For this review, take the finished solid that the model builds, in its own axes (mm). A direction names the side the tool comes from. Coordinates: 2 decimals unless noted, no trailing zeros. Loops run counter-clockwise (first coordinate to the right, second up) from the corner with the lowest first, then second, coordinate; pieces in that order, holes last.
1. Machinability: for faces 4 (the face through (2, -5, 5)), 5 (the face through (2, 7, 0)), which of the approach directions +Z, -Z, +X, -X, +Y, -Y give a long, thin tool a straight path to every point of the face, cutting with its end or side? Answer none if there is none.
2. Clearance check with flat-ended pins moving along their axes: P1, Ø2.5, axis at x = 12, z = 5, coming from the +Y side; P2, Ø4, axis at y = 1, z = 8.5, coming from the -X side; P3, Ø1.8, axis at x = 12, z = 5, coming from the -Y side. State where each tip first meets the part, or that it passes through.
3. Take a section at D-D, the plane y = -4.25. State the section outline as (x, z) points.
4. Take a section at A-A, the plane x = 3. State the section outline as (y, z) points.
5. Mouldability with a two-part tool opening along Y and no side actions: class faces 1 (the face through (13, 0, 5)), 2 (the face through (2, -10, 5)), 3 (the face through (3, 10, 5)) as pulls with the +Y half, pulls with the -Y half, needs draft (parallel to the pull), parting line crosses it, or undercut.
6. To check wall thickness, follow probe 1 along X at (y, z) = (8.1, 5); probe 2 along Y at (x, z) = (12.75, 6.25); probe 3 along Z at (x, y) = (12, -6.45). State the ranges of each line that lie inside material, in increasing order.
7. Take a section at C-C, the plane y = -7.5. State the section outline as (x, z) points, then the cut area to 3 significant figures.
8. Take a section at B-B, the plane z = 7. State the section outline as (x, y) points.
```python
from build123d import *

# Parameters (mm, degrees)
F0_W     = 2
F0_H     = 10
F1_DEPTH = 10
F3_DEPTH = 20


with BuildPart() as f1:
    # F0 (on Top) → F1 (new body)
    with BuildSketch(Plane.XY):
        Polygon((-1, 5), (0, 5), (1, 5), (13, 5), (15, 5), (15, 10), (-10, 10), (-10, 5), align=None)
        Polygon((1, -5), (0, -5), (-1, -5), (-10, -5), (-10, -10), (15, -10), (15, -5), (13, -5), align=None)
        with Locations((14, 0)):
            Rectangle(F0_W, F0_H)
    extrude(amount=F1_DEPTH)

    # F2 (on face) → F3 (cut)
    with BuildSketch(Plane.XZ.offset(10)):
        with BuildLine():
            ThreePointArc((12, 4), (12.707107, 4.292893), (13, 5))
            ThreePointArc((13, 5), (11.292893, 5.707107), (12, 4))
        make_face()
        with BuildLine():
            ThreePointArc((-7, 4), (-6.292893, 4.292893), (-6, 5))
            ThreePointArc((-6, 5), (-7.707107, 5.707107), (-7, 4))
        make_face()
    extrude(amount=-F3_DEPTH, mode=Mode.SUBTRACT)


solid = f1.part
```
Results list:
1. face 4: +Z, -Z, -X
1. face 5: -Z, +X, -X, +Y, -Y
2. P1: stops at y = 10
2. P2: stops at x = 13
2. P3: passes through
3. outline: (13, 0) - (15, 0) - (15, 10) - (13, 10) - close
4. outline: (-10, 0) - (-5, 0) - (-5, 10) - (-10, 10) - close; (5, 0) - (10, 0) - (10, 10) - (5, 10) - close
5. face 1: undercut
5. face 2: pulls with the -Y half
5. face 3: pulls with the +Y half
6. probe 1: x = -10 to -8, -6 to 11, 13 to 15
6. probe 2: y = -10 to -5, 5 to 10
6. probe 3: z = 0 to 4, 6 to 10
7. outline: (-10, 0) - (15, 0) - (15, 10) - (-10, 10) - close; hole circle Ø2 at (-7, 5); hole circle Ø2 at (12, 5)
7. area: 244 mm2
8. outline: (-10, -10) - (15, -10) - (15, 10) - (-10, 10) - (-10, 5) - (13, 5) - (13, -5) - (-10, -5) - close
